Source: CAD feature listing. Evaluate the final solid. Frame: model axes, mm. Coordinates: 2 decimals unless noted, no trailing zeros. Write each loop counter-clockwise with the first axis right and the second up, starting at its lowest first coordinate (ties: lowest second). Pieces come first, ordered by that corner, then holes. Notation, with made-up numbers: (41, 37) - (85, 37) arc R22 cw to (85, 60) - close; hole circle Ø4 at (75.25, 62). An arc over 180 degrees is marked (long way). One line per question, with ' | ' between items. Start each with the question number.
Q1. Cut plane C-C, the plane x = -457. Return loops of the section in (y, z).
Q2. Line query: line 1 (Z direction, x = -360, y = 4.5); line 2 (Y direction, x = -392, z = 0); line 3 (Y direction, x = -173, z = 47). Output: solid intervals per line, ascending.
Q3. Contact query for flat-ended pins moving along their axis: P1, Ø10, axis at x = -659, z = 42.5, coming from the +Y side; P2, Ø4, axis at x = -292.5, z = 129.5, coming from the -Y side; P3, Ø2, axis at x = -166.5, y = -4.5, coming from the -Z side. Output: stop coordinate, or through.
Q4. Draft query along Z for faces 1 (the face through (-369.778, -153.755, 34.143)), 2 (the face through (0, -157, -36)), 3 (the face through (-369.778, -161.564, 35.877)). Return one class per face: +Z half, -Z half, draft (parallel to the pull), parting line (faces both ways), or undercut.
Q5. Cut plane A-A, the plane y = 0. Return loops of the section in (x, z), plus the area to 3 significant figures.
```python
from build123d import *

# Parameters (mm, degrees)
SKETCH1_R           = 165.5
BOSS_EXTRUDE1_DEPTH = 750
SKETCH2_R           = 157.5
CUT_EXTRUDE1_DEPTH  = 750
FILLET1_R           = 2
FILLET2_R           = 2


with BuildPart() as part:
    # Sketch1 → Boss-Extrude1 (new body)
    with BuildSketch(Plane(origin=(0, 0, 0), x_dir=(0, 0, -1), z_dir=(1, 0, 0))):
        Circle(SKETCH1_R)
    extrude(amount=-BOSS_EXTRUDE1_DEPTH)

    # Sketch2 → Cut-Extrude1 (cut)
    with BuildSketch(Plane(origin=(0, 0, 0), x_dir=(0, 0, -1), z_dir=(1, 0, 0))):
        Circle(SKETCH2_R)
    extrude(amount=-CUT_EXTRUDE1_DEPTH, mode=Mode.SUBTRACT)

    # Fillet1
    fillet1_edges = [part.edges().sort_by_distance(p)[0] for p in [
        (0, 0, 165.5),
        (0, 0, 157.5),
    ]]
    fillet(fillet1_edges, radius=FILLET1_R)

    # Fillet2
    fillet2_edges = [part.edges().sort_by_distance(p)[0] for p in [
        (-750, 0, 165.5),
        (-750, 0, 157.5),
    ]]
    fillet(fillet2_edges, radius=FILLET2_R)


solid = part.part
```
Reply:
1) outline: circle Ø331 at (0, 0); hole circle Ø315 at (0, 0)
2) line 1: z = -165.44 to -157.44, 157.44 to 165.44 | line 2: y = -165.5 to -157.5, 157.5 to 165.5 | line 3: y = -158.69 to -150.32, 150.32 to 158.69
3) P1: stops at y = 161.2 | P2: stops at y = -105.52 | P3: stops at z = -165.46
4) face 1: undercut | face 2: draft | face 3: parting line
5) outline: (-750, -163.5) arc R2 ccw to (-748, -165.5) - (-2, -165.5) arc R2 ccw to (0, -163.5) - (0, -159.5) arc R2 ccw to (-2, -157.5) - (-748, -157.5) arc R2 ccw to (-750, -159.5) - close; (-750, 159.5) arc R2 ccw to (-748, 157.5) - (-2, 157.5) arc R2 ccw to (0, 159.5) - (0, 163.5) arc R2 ccw to (-2, 165.5) - (-748, 165.5) arc R2 ccw to (-750, 163.5) - close | area: 12,000 mm^2
